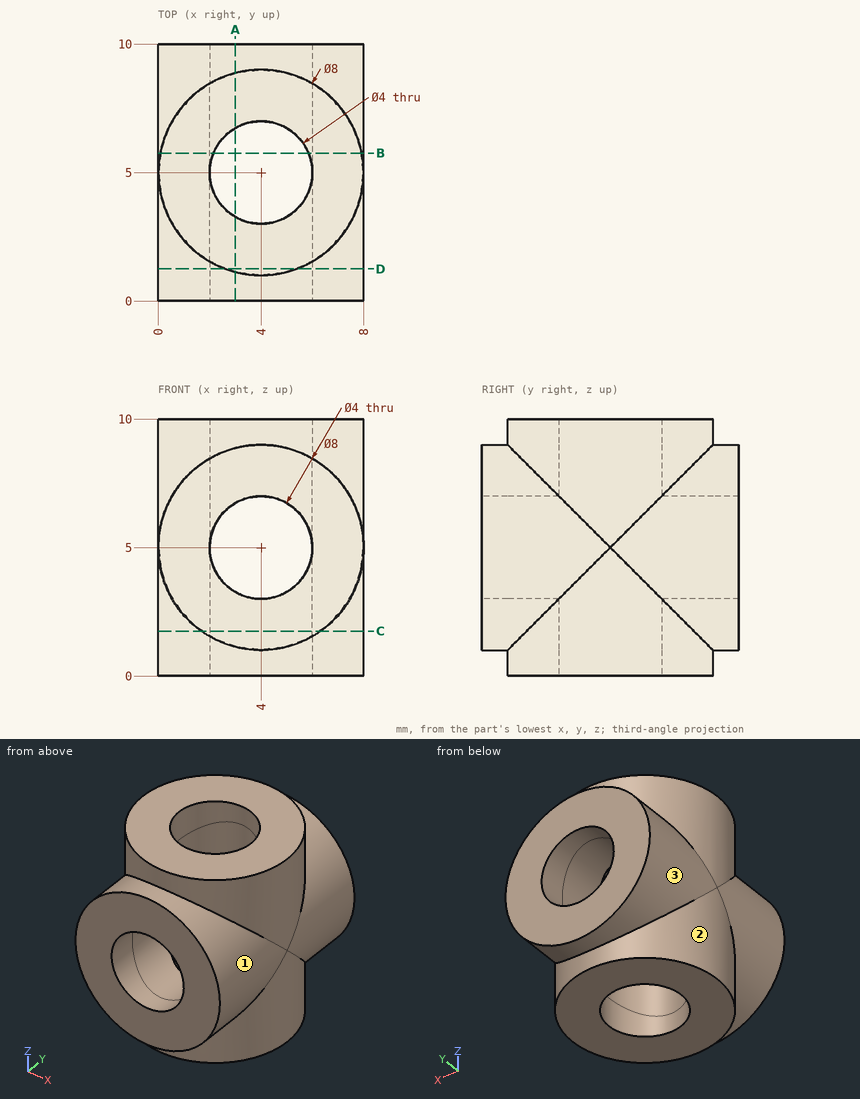
Geometry: see drawing. Coordinates: mm, zero at the bounding-box minimum. A direction names the side the tool comes from. Coordinates: 2 decimals unless noted, no trailing zeros. Order: outer loops, then holes, each group sorted by start corner. A loop starts at its lowest first (then second) coordinate and runs counter-clockwise, first axis right, second up. Notation, with made-up numbers: M 9,82 L 44,82 A7 cw 44,91 Z; hole C 56,-20 d1. An arc over 180 degrees is marked long. Write each question's results on one line, items separated by ' | '. Start each with the question number.
1) Section query C-C (z = 1.75). Return the cut outline in (x, y).
2) Line query: line 1 (Y direction, x = 4, z = 1.95); line 2 (Z direction, x = 4, y = 9.1). Output: solid intervals per line, ascending. Write a range as from..to.
3) Contact query for flat-ended pins moving along their axis: pin 1 Ø3 at (x, z) = (5, 6.5) entering from -Y; pin 2 Ø1 at (y, z) = (2.5, 1.5) entering from -X. Output: stop coordinate, or through.
4) Section query A-A (x = 3). Return the cut outline in (y, z), plus the area to 3 significant figures.
5) Access query for the marked faces 1, 2 and 3. Directions: +Z, -Z, +X, -X, +Y, -Y. A direction counts if a zero-diameter tool reaches every point of the face in a straight line with its end or side. Return the directions, or none.
6) Section query B-B (y = 5.75). Return the cut outline in (x, z).
7) Section query D-D (y = 1.25). Return the cut outline in (x, z), plus the area to 3 significant figures.
Answers:
1) outline: M 1.67,0 L 6.33,0 L 6.33,1.75 A4 ccw 6.33,8.25 L 6.33,10 L 1.67,10 L 1.67,8.25 A4 ccw 1.67,1.75 Z; hole C 4,5 d4
2) line 1: y = 0..3, 7..10 | line 2: z = 1..3, 7..9
3) pin 1: stops at y = 0 | pin 2: stops at x = 0.54
4) outline: M 0,1.13 L 1.13,1.13 L 1.13,0 L 3.27,0 L 3.27,3.27 L 0,3.27 Z; M 0,6.73 L 3.27,6.73 L 3.27,10 L 1.13,10 L 1.13,8.87 L 0,8.87 Z; M 6.73,0 L 8.87,0 L 8.87,1.13 L 10,1.13 L 10,3.27 L 6.73,3.27 Z; M 6.73,6.73 L 10,6.73 L 10,8.87 L 8.87,8.87 L 8.87,10 L 6.73,10 Z | area: 37.6 mm^2
5) face 1: -Y | face 2: -Z | face 3: +Y
6) outline: M 0.07,0 L 2.15,0 L 2.15,4.25 A2 cw 2.15,5.75 L 2.15,10 L 0.07,10 L 0.07,5.75 A4 ccw 0.07,4.25 Z; M 5.85,0 L 7.93,0 L 7.93,4.25 A4 ccw 7.93,5.75 L 7.93,10 L 5.85,10 L 5.85,5.75 A2 cw 5.85,4.25 Z
7) outline: M 2.61,0 L 5.39,0 L 5.39,1.25 A4 ccw 5.39,8.75 L 5.39,10 L 2.61,10 L 2.61,8.75 A4 ccw 2.61,1.25 Z; hole C 4,5 d4 | area: 43.7 mm^2
